Check sheet for the modelled part. Datum: model origin and axes. Units: mm. Face numbers are marked on the shaded views. A direction names the side the tool comes from. Give positions to 0.01 mm unless a question says otherwise; leave off trailing zeros. Order: outer loops, then holes, each group sorted by start corner. A loop starts at its lowest first (then second) coordinate and runs counter-clockwise, first axis right, second up.
```python
from build123d import *

# Parameters (mm, degrees)
SKETCH1_W           = 80
SKETCH1_H           = 54
BOSS_EXTRUDE1_DEPTH = 30
SKETCH2_W           = 76
SKETCH2_H           = 50
CUT_EXTRUDE1_DEPTH  = 28
CUT_EXTRUDE2_DEPTH  = 6
SKETCH4_W           = 36
SKETCH4_H           = 18
CUT_EXTRUDE3_DEPTH  = 6
SKETCH5_W           = 2.5
SKETCH5_H           = 2.5
STANDOFFS_DEPTH     = 4
FILLET3_R           = 9
FILLET4_R           = 9
SKETCH6_W           = 3
SKETCH6_H           = 45
BOTTOM_GRILL_DEPTH  = 2
CUT_EXTRUDE5_REACH  = 75.593
SKETCH7_W           = 2
SKETCH7_H           = 22
CUT_EXTRUDE6_START  = -54
SKETCH8_R           = 1.75
CUT_EXTRUDE6_DEPTH  = 54
SKETCH9_R           = 1.75
CUT_EXTRUDE7_DEPTH  = 2


with BuildPart() as part:
    # Sketch1 → Boss-Extrude1 (new body)
    with BuildSketch(Plane(origin=(0, 0, 0), x_dir=(1, 0, 0), z_dir=(0, 1, 0))):
        Rectangle(SKETCH1_W, SKETCH1_H)
    extrude(amount=BOSS_EXTRUDE1_DEPTH)

    # Sketch2 → Cut-Extrude1 (cut)
    with BuildSketch(Plane(origin=(0, 30, 0), x_dir=(1, 0, 0), z_dir=(0, 1, 0))):
        Rectangle(SKETCH2_W, SKETCH2_H)
    extrude(amount=-CUT_EXTRUDE1_DEPTH, mode=Mode.SUBTRACT)

    # Sketch3 → Cut-Extrude2 (cut)
    with BuildSketch(Plane(origin=(40, 0, 0), x_dir=(0, 0, -1), z_dir=(1, 0, 0))):
        with BuildLine():
            Line((5.5, 15), (5.5, 5))
            Line((5.5, 5), (-9.5, 5))
            Line((-9.5, 5), (-9.5, 15))
            ThreePointArc((-9.5, 15), (-2, 22.5), (5.5, 15))
        make_face()
    extrude(amount=-CUT_EXTRUDE2_DEPTH, mode=Mode.SUBTRACT)

    # Sketch4 → Cut-Extrude3 (cut)
    with BuildSketch(Plane.ZY.offset(40)):
        with Locations((0, 20)):
            Rectangle(SKETCH4_W, SKETCH4_H)
    extrude(amount=-CUT_EXTRUDE3_DEPTH, mode=Mode.SUBTRACT)

    # Sketch5 → Standoffs (add)
    with BuildSketch(Plane(origin=(0, 2, 0), x_dir=(1, 0, 0), z_dir=(0, 1, 0))):
        with Locations((36.75, 23.75)):
            Rectangle(SKETCH5_W, SKETCH5_H)
        with Locations((36.75, -23.75)):
            Rectangle(SKETCH5_W, SKETCH5_H)
        with Locations((-36.75, -23.75)):
            Rectangle(SKETCH5_W, SKETCH5_H)
        with Locations((-36.75, 23.75)):
            Rectangle(SKETCH5_W, SKETCH5_H)
    extrude(amount=STANDOFFS_DEPTH)

    # Fillet3
    fillet3_edges = [part.edges().sort_by_distance(p)[0] for p in [
        (-39, 29, -18),
    ]]
    fillet(fillet3_edges, radius=FILLET3_R)

    # Fillet4
    fillet4_edges = [part.edges().sort_by_distance(p)[0] for p in [
        (-39, 29, 18),
    ]]
    fillet(fillet4_edges, radius=FILLET4_R)

    # Sketch6 → Bottom Grill (cut)
    with BuildSketch(Plane.XZ):
        with Locations((33.5, 0)):
            Rectangle(SKETCH6_W, SKETCH6_H)
        with Locations((24.5, 0)):
            Rectangle(SKETCH6_W, SKETCH6_H)
        with Locations((15.5, 0)):
            Rectangle(SKETCH6_W, SKETCH6_H)
        with Locations((6.5, 0)):
            Rectangle(SKETCH6_W, SKETCH6_H)
        with Locations((-2.5, 0)):
            Rectangle(SKETCH6_W, SKETCH6_H)
        with Locations((-11.5, 0)):
            Rectangle(SKETCH6_W, SKETCH6_H)
    extrude(amount=-BOTTOM_GRILL_DEPTH, mode=Mode.SUBTRACT)

    # Cut-Extrude5: up to this face of the body (flat: up to its plane)
    cut_extrude5_end = Plane(part.part.faces().sort_by_distance((0, 15, 27))[0])
    # Sketch7 → Cut-Extrude5 (cut, up to the picked face)
    with BuildSketch(Plane(origin=(0, 0, -27), x_dir=(-1, 0, 0), z_dir=(0, 0, -1)), mode=Mode.PRIVATE) as cut_extrude5_sk1:
        with Locations((-33, 15)):
            Rectangle(SKETCH7_W, SKETCH7_H)
    cut_extrude5_tool1 = split(extrude(cut_extrude5_sk1.sketch, amount=-CUT_EXTRUDE5_REACH, mode=Mode.PRIVATE), bisect_by=cut_extrude5_end, keep=Keep.BOTH, mode=Mode.PRIVATE)
    # Sketch7 → Cut-Extrude5 (cut, up to the picked face)
    with BuildSketch(Plane(origin=(0, 0, -27), x_dir=(-1, 0, 0), z_dir=(0, 0, -1)), mode=Mode.PRIVATE) as cut_extrude5_sk2:
        with Locations((-25, 15)):
            Rectangle(SKETCH7_W, SKETCH7_H)
    cut_extrude5_tool2 = split(extrude(cut_extrude5_sk2.sketch, amount=-CUT_EXTRUDE5_REACH, mode=Mode.PRIVATE), bisect_by=cut_extrude5_end, keep=Keep.BOTH, mode=Mode.PRIVATE)
    # Sketch7 → Cut-Extrude5 (cut, up to the picked face)
    with BuildSketch(Plane(origin=(0, 0, -27), x_dir=(-1, 0, 0), z_dir=(0, 0, -1)), mode=Mode.PRIVATE) as cut_extrude5_sk3:
        with Locations((-17, 15)):
            Rectangle(SKETCH7_W, SKETCH7_H)
    cut_extrude5_tool3 = split(extrude(cut_extrude5_sk3.sketch, amount=-CUT_EXTRUDE5_REACH, mode=Mode.PRIVATE), bisect_by=cut_extrude5_end, keep=Keep.BOTH, mode=Mode.PRIVATE)
    # Sketch7 → Cut-Extrude5 (cut, up to the picked face)
    with BuildSketch(Plane(origin=(0, 0, -27), x_dir=(-1, 0, 0), z_dir=(0, 0, -1)), mode=Mode.PRIVATE) as cut_extrude5_sk4:
        with Locations((-9, 15)):
            Rectangle(SKETCH7_W, SKETCH7_H)
    cut_extrude5_tool4 = split(extrude(cut_extrude5_sk4.sketch, amount=-CUT_EXTRUDE5_REACH, mode=Mode.PRIVATE), bisect_by=cut_extrude5_end, keep=Keep.BOTH, mode=Mode.PRIVATE)
    # Sketch7 → Cut-Extrude5 (cut, up to the picked face)
    with BuildSketch(Plane(origin=(0, 0, -27), x_dir=(-1, 0, 0), z_dir=(0, 0, -1)), mode=Mode.PRIVATE) as cut_extrude5_sk5:
        with Locations((-1, 15)):
            Rectangle(SKETCH7_W, SKETCH7_H)
    cut_extrude5_tool5 = split(extrude(cut_extrude5_sk5.sketch, amount=-CUT_EXTRUDE5_REACH, mode=Mode.PRIVATE), bisect_by=cut_extrude5_end, keep=Keep.BOTH, mode=Mode.PRIVATE)
    # Sketch7 → Cut-Extrude5 (cut, up to the picked face)
    with BuildSketch(Plane(origin=(0, 0, -27), x_dir=(-1, 0, 0), z_dir=(0, 0, -1)), mode=Mode.PRIVATE) as cut_extrude5_sk6:
        with Locations((7, 15)):
            Rectangle(SKETCH7_W, SKETCH7_H)
    cut_extrude5_tool6 = split(extrude(cut_extrude5_sk6.sketch, amount=-CUT_EXTRUDE5_REACH, mode=Mode.PRIVATE), bisect_by=cut_extrude5_end, keep=Keep.BOTH, mode=Mode.PRIVATE)
    add(cut_extrude5_tool1.solids().sort_by(Axis((33, 15, -27), (0, 0, 1)))[0], mode=Mode.SUBTRACT)
    add(cut_extrude5_tool2.solids().sort_by(Axis((25, 15, -27), (0, 0, 1)))[0], mode=Mode.SUBTRACT)
    add(cut_extrude5_tool3.solids().sort_by(Axis((17, 15, -27), (0, 0, 1)))[0], mode=Mode.SUBTRACT)
    add(cut_extrude5_tool4.solids().sort_by(Axis((9, 15, -27), (0, 0, 1)))[0], mode=Mode.SUBTRACT)
    add(cut_extrude5_tool5.solids().sort_by(Axis((1, 15, -27), (0, 0, 1)))[0], mode=Mode.SUBTRACT)
    add(cut_extrude5_tool6.solids().sort_by(Axis((-7, 15, -27), (0, 0, 1)))[0], mode=Mode.SUBTRACT)

    # Sketch8 → Cut-Extrude6 (cut)
    with BuildSketch(Plane(origin=(0, 0, -27), x_dir=(-1, 0, 0), z_dir=(0, 0, -1)).offset(CUT_EXTRUDE6_START)):
        with Locations((-13, 27)):
            Circle(SKETCH8_R)
        with Locations((25, 27)):
            Circle(SKETCH8_R)
    extrude(amount=CUT_EXTRUDE6_DEPTH, mode=Mode.SUBTRACT)

    # Sketch9 → Cut-Extrude7 (cut)
    with BuildSketch(Plane.ZY.offset(40)):
        with Locations((-23, 26)):
            Circle(SKETCH9_R)
        with Locations((23, 26)):
            Circle(SKETCH9_R)
    extrude(amount=-CUT_EXTRUDE7_DEPTH, mode=Mode.SUBTRACT)


solid = part.part
```
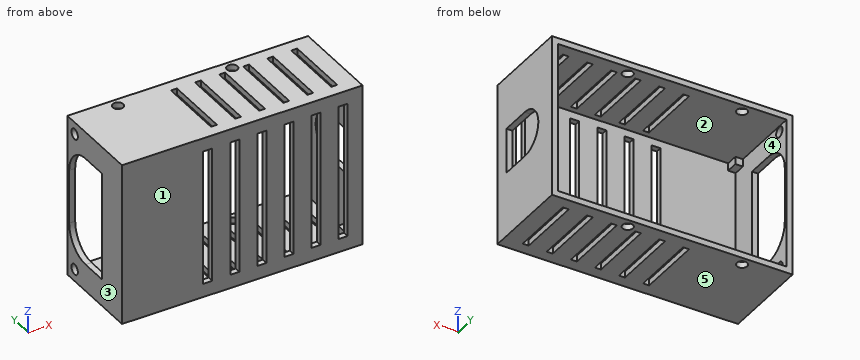
(1) Gauge pin test, flat ends, axial feed: pin 1 Ø2 at (x, z) = (0, 15) entering from +Y; pin 2 Ø3 at (x, y) = (13, 27) entering from +Z. Record the tip position at first contact, or that the pin passes through.
Response values:
pin 1: stops at y = 2
pin 2: passes through
(2) Set-up check for the marked faces 4 and 5: record each of +Z, -Z, +X, -X, +Y, -Y from which the full face is reachable in a straight line by a thin tool's end or side.
Response values:
face 4: +Y
face 5: -Z, +X, -X, +Y, -Y
(3) Cross-section at B-B on x = -25. Enter the section's corners in (y, z), then the cut area to 3 significant figures.
Response values:
outline: (0, -27) - (25.25, -27) - (25.25, -25) - (2, -25) - (2, 25) - (25.25, 25) - (25.25, 27) - (0, 27) - close; (28.75, -27) - (30, -27) - (30, -25) - (28.75, -25) - close; (28.75, 25) - (30, 25) - (30, 27) - (28.75, 27) - close
area: 206 mm2
(4) Cross-section at D-D on x = 30.5. Enter the section's corners in (y, z), then the cut area to 3 significant figures.
Response values:
outline: (0, -27) - (30, -27) - (30, -25) - (2, -25) - (2, 25) - (30, 25) - (30, 27) - (0, 27) - close
area: 220 mm2
(5) Cross-section at A-A on z = -19. Count the separate pieces of the cut face and the enclosed holes in it, then the cut area to 3 significant figures.
Response values:
separate pieces: 7
enclosed holes: 0
area: 236 mm2
(6) Release check for a two-part mould opening along X. For the marked faces 1, 2 and 3 record: released by +X, released by -X, zero draft, split by the parting line, or undercut.
Response values:
face 1: zero draft
face 2: undercut
face 3: released by -X
(7) Material ranges on L1, parallel to X at y = 27, z = -26.5; L2, parallel to Z at x = 6.5, y = 6.25; L3, parallel to Y at x = -38.6, z = 23, recorded low to high.
Response values:
L1: x = -40 to -26.75, -23.25 to 11.25, 14.75 to 40
L2: z = -27 to -25, 25 to 27
L3: y = 0 to 24.25, 27.75 to 30
